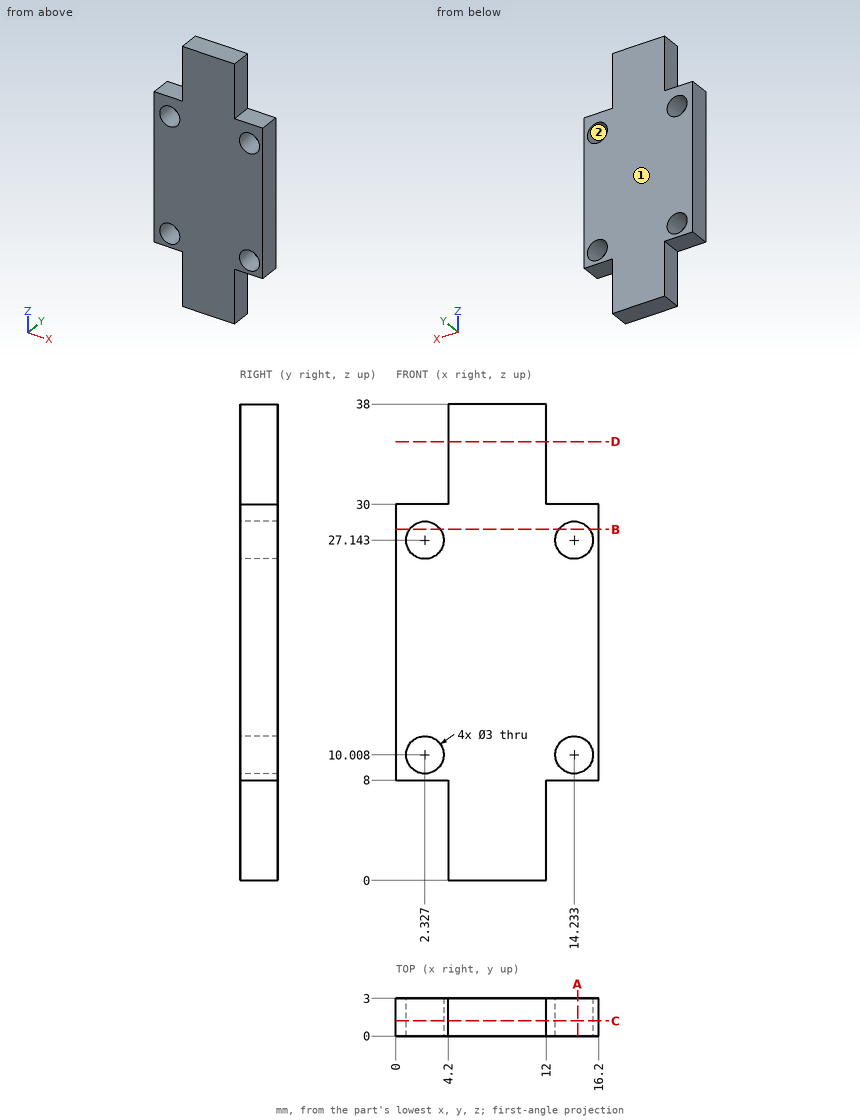
The figure shows three views and two pictorial views of one solid part (mm, origin at its lowest corner). Answer the questions. Coordinates: 2 decimals unless noted, no trailing zeros. Loops run counter-clockwise (first coordinate to the right, second up) from the corner with the lowest first, then second, coordinate; pieces in that order, holes last. Notation, with made-up numbers: M 39.25,18 L 52.25,18 A27 cw 52.25,34 Z; hole C -20.5,19 d10. An arc over 180 degrees is marked long. Use CSV: the item, a comma, the result in double quotes. Start each with the question number.
(1) Consider line 1 (Z direction, x = 15, y = 2.55) (1 decimal); line 2 (Z direction, x = 13, y = 1.8) (1 decimal); line 3 (X direction, y = 1.55, z = 3). Determine where each line is inside the solid, lowest interval first.
(2) Find section C-C, the plane y = 1.2. Give the vertices of the cut face in (x, z), then the cut area to 3 significant figures.
(3) Find section B-B, the plane z = 28. Give the vertices of the cut face in (x, y) (1 decimal).
(4) For a pull along X with two mould halves and no side action, classify the marked faces 1 and 2 as +X half, -X half, draft (parallel to the pull), parting line (faces both ways), or undercut.
(5) Given pin 1 Ø0.9 at (x, y) = (14, 1) entering from +Z; pin 2 Ø1.5 at (x, y) = (1.5, 2) entering from -Z; pin 3 Ø8 at (x, z) = (12.5, 4) entering from +Y; pin 4 Ø1.5 at (y, z) = (2, 33) entering from -X, each flat-ended and moving along its own axis, determine where each tip first touches the part or whether it passes through.
(6) Find section A-A, the plane x = 14.5. Give the vertices of the cut face in (y, z).
(7) Find section D-D, the plane z = 35. Give the vertices of the cut face in (x, y), then the cut area to 3 significant figures.
Recorded:
1,line 1,"z = 8 to 8.7, 11.3 to 25.9, 28.4 to 30"
1,line 2,"z = 8 to 9.2, 10.9 to 26.3, 28 to 30"
1,line 3,"x = 4.2 to 12"
2,outline,"M 0,8 L 4.2,8 L 4.2,0 L 12,0 L 12,8 L 16.2,8 L 16.2,30 L 12,30 L 12,38 L 4.2,38 L 4.2,30 L 0,30 Z; hole C 2.33,10.01 d3; hole C 2.33,27.14 d3; hole C 14.23,10.01 d3; hole C 14.23,27.14 d3"
2,area,"453 mm^2"
3,outline,"M 0,0 L 1.1,0 L 1.1,3 L 0,3 Z; M 3.6,0 L 13,0 L 13,3 L 3.6,3 Z; M 15.5,0 L 16.2,0 L 16.2,3 L 15.5,3 Z"
4,face 1,"draft"
4,face 2,"undercut"
5,pin 1,"stops at z = 30"
5,pin 2,"stops at z = 8"
5,pin 3,"stops at y = 3"
5,pin 4,"stops at x = 4.2"
6,outline,"M 0,8 L 3,8 L 3,8.53 L 0,8.53 Z; M 0,11.48 L 3,11.48 L 3,25.67 L 0,25.67 Z; M 0,28.62 L 3,28.62 L 3,30 L 0,30 Z"
7,outline,"M 4.2,0 L 12,0 L 12,3 L 4.2,3 Z"
7,area,"23.4 mm^2"
